from build123d import *

# Parameters (mm, degrees)
SKETCH046_R     = 2
PAD031_DEPTH    = 3
PAD032_DEPTH    = 121
SKETCH048_R     = 2
POCKET006_DEPTH = 5
PAD034_DEPTH    = 5
PAD035_DEPTH    = 2


with BuildPart() as part:
    # Sketch046 → Pad031 (new body)
    with BuildSketch(Plane.XZ):
        with BuildLine():
            Line((-97.078247, 0), (24.252445, 0))
            Line((24.252445, 31.132916), (24.252445, 0))
            ThreePointArc((24.252445, 31.132916), (23.699133, 32.468728), (22.363321, 33.02204))
            Line((10.487469, 33.02204), (22.363321, 33.02204))
            ThreePointArc((10.487469, 33.02204), (8.798373, 32.322393), (8.098726, 30.633297))
            Line((8.098726, 20.736529), (8.098726, 30.633297))
            ThreePointArc((-4.637803, 8), (4.368283, 11.730443), (8.098726, 20.736529))
            Line((-24.402262, 8), (-4.637803, 8))
            ThreePointArc((-28.139309, 11.737048), (-27.044753, 9.094556), (-24.402262, 8))
            Line((-28.139309, 13.595442), (-28.139309, 11.737048))
            ThreePointArc((-28.139309, 13.595442), (-28.619727, 14.755273), (-29.779558, 15.235691))
            Line((-38.786943, 15.235691), (-29.779558, 15.235691))
            ThreePointArc((-38.786943, 15.235691), (-39.805693, 14.813711), (-40.227672, 13.794961))
            Line((-40.227672, 11.868778), (-40.227672, 13.794961))
            ThreePointArc((-44.096451, 8), (-41.360811, 9.133139), (-40.227672, 11.868778))
            Line((-66.045778, 8), (-44.096451, 8))
            ThreePointArc((-79.770671, 21.724892), (-75.750743, 12.019928), (-66.045778, 8))
            Line((-79.770671, 37.210011), (-79.770671, 21.724892))
            ThreePointArc((-79.770671, 37.210011), (-80.669155, 39.379145), (-82.838289, 40.277629))
            Line((-91.200258, 40.277629), (-82.838289, 40.277629))
            ThreePointArc((-91.200258, 40.277629), (-92.81323, 39.609514), (-93.481345, 37.996542))
            Line((-93.481345, 10.816122), (-93.481345, 37.996542))
            ThreePointArc((-96.297467, 8), (-94.306168, 8.824823), (-93.481345, 10.816122))
            Line((-97.078247, 8), (-96.297467, 8))
            Line((-97.078247, 0), (-97.078247, 8))
        make_face()
        with Locations((-86, 36.5)):
            Circle(SKETCH046_R, mode=Mode.SUBTRACT)
        with Locations((-86, 11.5)):
            Circle(SKETCH046_R, mode=Mode.SUBTRACT)
        with Locations((-34, 11.5)):
            Circle(SKETCH046_R, mode=Mode.SUBTRACT)
        with Locations((19, 30.5)):
            Circle(SKETCH046_R, mode=Mode.SUBTRACT)
        with Locations((19, 11.5)):
            Circle(SKETCH046_R, mode=Mode.SUBTRACT)
    extrude(amount=PAD031_DEPTH)

    # Sketch047 → Pad032 (join)
    with BuildSketch(Plane.YZ.offset(24)):
        Polygon((-3, 0), (-16, 0), (-16, 3), (-6, 3), (-3, 7.999382), align=None)
    extrude(amount=-PAD032_DEPTH)

    # Sketch048 → Pocket006 (cut)
    with BuildSketch(Plane.XY):
        with Locations((-64, -11)):
            Circle(SKETCH048_R)
        with Locations((0, -11)):
            Circle(SKETCH048_R)
    extrude(amount=POCKET006_DEPTH, mode=Mode.SUBTRACT)

    # Sketch054 → Pad034 (join)
    with BuildSketch(Plane.YZ.offset(9)):
        Polygon((-2.747999, 30.548568), (-2.747999, 16.500504), (-8.678396, 2.710541), (-15.46899, 2.710541), align=None)
    extrude(amount=PAD034_DEPTH)

    # Sketch055 → Pad035 (join)
    with BuildSketch(Plane.YZ.offset(-93)):
        Polygon((-2.747999, 30.548568), (-2.747999, 16.500504), (-8.678396, 2.710541), (-15.46899, 2.710541), align=None)
    extrude(amount=PAD035_DEPTH)


with BuildPart() as part_1:
    # Body011 placement: moved
    add(part.part.moved(Location((0, -18, -41.5))))


solid = part_1.part
Work out the finished part from the listing and answer in its coordinate system (mm). A direction names the side the tool comes from. Coordinates: 2 decimals unless noted, no trailing zeros. Loops run counter-clockwise (first coordinate to the right, second up) from the corner with the lowest first, then second, coordinate; pieces in that order, holes last. Notation, with made-up numbers: (76, 37.5) -> (109, 37.5) arc R18 ccw to (109, 60.5) -> close; hole circle Ø9 at (-21, -5). An arc over 180 degrees is marked (long way). Write each question's results on one line, items separated by ' | '. Start each with the question number.
1) Consider line 1 along Z through (x, y) = (19, -19.95); line 2 along X through (y, z) = (-29, -40.7); line 3 along X through (y, z) = (-21.75, -26). Determine where each line is inside the solid, lowest interval first.
2) Find section A-A on x = 19. Determine the outline of the cut face in (y, z).
3) Find section D-D on x = -34. Determine the outline of the cut face in (y, z).
4) For faces 1 (the cylindrical face through (-27.07, -19.48, -32.38)), 2 (the flat face through (16, -19, -8.478)), 3 (the flat face through (14, -27, -29)), determine the directions among +Z, -Z, +X, -X, +Y, -Y from which every point of the face is accessible in a straight line to the end or side of a thin tool.
5) Find section C-C on y = -19.5. Count the separate pieces of the cut face and the enclosed holes in it, then the cut area to 3 significant figures.
6) Flat-ended cylindrical pins translate along their axes: P1, Ø4, axis at y = -26, z = -39, coming from the +X side; P2, Ø1.5, axis at x = -36.5, y = -19, coming from the +Z side; P3, Ø2, axis at y = -23, z = -16, coming from the -X side; P4, Ø4.5, axis at x = 19, z = -30, coming from the +Y side. Find the tip coordinate at first contact, or state that the pin passes through.
7) Find section B-B on z = -35. Determine the outline of the cut face in (x, y).
8) The mould has two halves that part along X. Classify faces 4 (the cylindrical face through (19, -19, -32)), 5 (the flat face through (-93.481, -19, -17)), 6 (the cylindrical face through (-64, -31, -40)), 7 (the flat face through (-35.7, -22.5, -36)): pulls with the +X half, pulls with the -X half, needs draft (parallel to the pull), parting line crosses it, or undercut.
Response values:
1) line 1: z = -41.5 to -32, -28 to -13, -9 to -8.48 | line 2: x = -97 to -66, -62 to -2, 2 to 24 | line 3: x = -93 to -91, 9 to 14
2) outline: (-34, -41.5) -> (-18, -41.5) -> (-18, -32) -> (-21, -32) -> (-21, -33.5) -> (-24, -38.5) -> (-34, -38.5) -> close; (-21, -28) -> (-18, -28) -> (-18, -13) -> (-21, -13) -> close; (-21, -9) -> (-18, -9) -> (-18, -8.48) -> (-21, -8.48) -> close
3) outline: (-34, -41.5) -> (-18, -41.5) -> (-18, -32) -> (-21, -32) -> (-21, -33.5) -> (-24, -38.5) -> (-34, -38.5) -> close; (-21, -28) -> (-18, -28) -> (-18, -26.26) -> (-21, -26.26) -> close
4) face 1: +Z, +Y, -Y | face 2: +Z, +X, +Y, -Y | face 3: +Z, +X, -Y
5) separate pieces: 1 | enclosed holes: 5 | area: 1,920 mm^2
6) P1: stops at x = 24 | P2: stops at z = -26.26 | P3: stops at x = -93 | P4: stops at y = -18
7) outline: (-97.08, -21) -> (-97, -21) -> (-97, -21.9) -> (24, -21.9) -> (24, -21) -> (24.25, -21) -> (24.25, -18) -> (-97.08, -18) -> close; (-93, -31.74) -> (-91, -31.74) -> (-91, -25.05) -> (-93, -25.05) -> close; (9, -31.74) -> (14, -31.74) -> (14, -25.05) -> (9, -25.05) -> close
8) face 4: undercut | face 5: pulls with the -X half | face 6: undercut | face 7: needs draft
